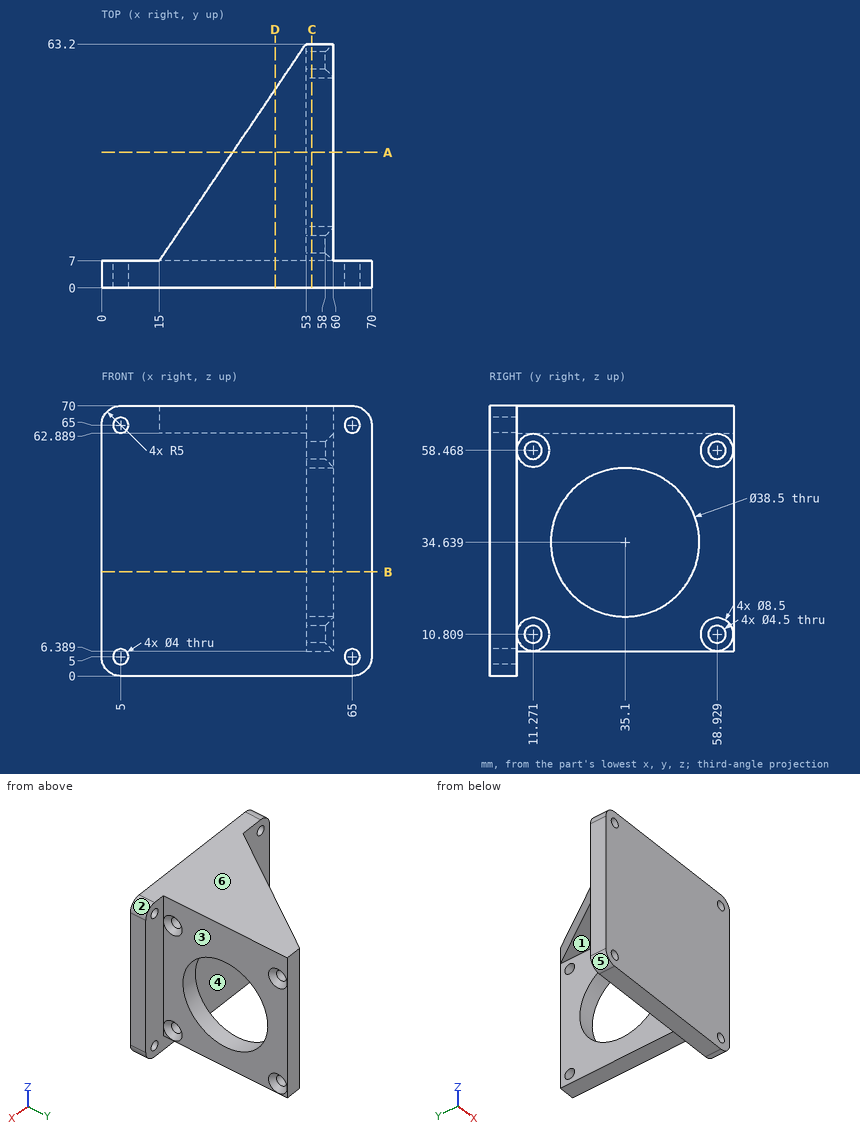
The figure shows three views and two pictorial views of one solid part (mm, origin at its lowest corner). Answer the questions. A direction names the side the tool comes from. Give positions to 0.01 mm unless a question says otherwise; leave off trailing zeros. Write each loop counter-clockwise with the first axis right and the second up, starting at its lowest first coordinate (ties: lowest second). Pieces come first, ordered by that corner, then holes.
Q1. A tool of negligible diameter and unlimited length cuts with its end or side. For the marked faces 1, 2 and 3, from which of +Z, -Z, +X, -X, +Y, -Y can it reach the whole face along a straight path? Write none if from no direction.
Answer:
face 1: -Z, -X, +Y
face 2: +Z, +X, +Y, -Y
face 3: +Z, -Z, +X, +Y
Q2. Straight lines are drawn through the part: L1, parallel to X at y = 4, z = 65; L2, parallel to Y at x = 55, z = 60 (1 decimal). For each, find the intervals that lie inside material, in ascending order.
Answer:
L1: x = 0 to 3, 7 to 63, 67 to 70
L2: y = 0 to 9.6, 12.9 to 57.3, 60.6 to 63.2
Q3. The part is cut by section D-D on x = 45. Give the vertices of the cut face in (y, z).
Answer:
outline: (0, 0) - (7, 0) - (7, 62.89) - (51.37, 62.89) - (51.37, 70) - (0, 70) - close
Q4. The part is cut by section B-B on z = 27. Give the vertices of the cut face in (x, y), and give its area (3 significant figures).
Answer:
outline: (0, 0) - (70, 0) - (70, 7) - (60, 7) - (60, 17.43) - (53, 17.43) - (53, 7) - (0, 7) - close; (53, 52.77) - (60, 52.77) - (60, 63.2) - (53, 63.2) - close
area: 636 mm2
Q5. For a pull along Z with two mould halves and no side action, classify the marked faces 4, 5 and 6 as released by +Z, released by -Z, zero draft, split by the parting line, or undercut.
Answer:
face 4: zero draft
face 5: released by -Z
face 6: released by +Z
Q6. The part is cut by section A-A on y = 35.1. Give the vertices of the cut face in (x, z), and give its area (3 significant figures).
Answer:
outline: (34, 62.89) - (53, 62.89) - (53, 53.89) - (60, 53.89) - (60, 70) - (34, 70) - close; (53, 6.39) - (60, 6.39) - (60, 15.39) - (53, 15.39) - close
area: 311 mm2
Q7. The part is cut by section C-C on x = 54.5. Give the vertices of the cut face in (y, z), and give its area (3 significant figures).
Answer:
outline: (0, 0) - (7, 0) - (7, 6.39) - (63.2, 6.39) - (63.2, 70) - (0, 70) - close; hole circle Ø4.5 at (11.27, 10.81); hole circle Ø4.5 at (11.27, 58.47); hole circle Ø38.5 at (35.1, 34.64); hole circle Ø4.5 at (58.93, 10.81); hole circle Ø4.5 at (58.93, 58.47)
area: 2,840 mm2
Q8. Given pin 1 (6.5 mm diameter, centred on x = 65, z = 5, fed in from -Y); pin 2 (7 mm diameter, centred on y = 58.93, z = 10.81, fed in from -X); pin 3 (2.5 mm diameter, centred on x = 5, z = 65, fed in from +Y); pin 4 (7.5 mm diameter, centred on x = 56, y = 44, fed in from -Z), each flat-ended and moving along its own axis, determine where each tip first touches the part or whether it passes through.
Answer:
pin 1: stops at y = 0
pin 2: stops at x = 53
pin 3: passes through
pin 4: stops at z = 6.39
